Here's how the part is built. I have some questions about the finished solid (model axes, mm). A direction names the side the tool comes from. Give positions to 0.01 mm unless a question says otherwise; leave off trailing zeros. Loops run counter-clockwise (first coordinate to the right, second up) from the corner with the lowest first, then second, coordinate; pieces in that order, holes last. Notation, with made-up numbers: (50, -0.75) -> (60, -0.75) arc R14 cw to (60, 3.25) -> close; hole circle Ø4 at (66.25, 13.25). An arc over 180 degrees is marked (long way). Answer in a Markdown table with one row per item. Add a question column.
Item 1: If we section it at D-D (x = -52): Write out the boundary of the cut face in (y, z), then the cut area to 3 significant figures.
Item 2: For P1, Ø5, axis at x = -53.5, z = 2, coming from the -Y side; P2, Ø3, axis at x = -10, z = 3, coming from the +Y side; P3, Ø2.5, axis at x = -5, z = 5, coming from the +Y side, each with a flat end and sliding along its axis, tell me the tip position at first contact or that it passes through.
Item 3: If I drill on line 1 (Z direction, x = -5, y = 3.5); line 2 (Y direction, x = -12.5, z = 8.5); line 3 (Z direction, x = -47.5, y = 5.75), over which ranges is the centre line in solid material (lowest first)?
Item 4: Which directions (+Z, -Z, +X, -X, +Y, -Y) give clear straight access to the entire face, cutting with the end or side of a thin tool? Please do faces 4 (the face through (0, 3, 5)), 5 (the face through (-18, 5, 5)).
Item 5: If we section it at C-C (z = 7.75): Write out the boundary of the cut face in (x, y).
Item 6: If we section it at A-A (x = -30): Write out the boundary of the cut face in (y, z).
Item 7: We'd pull the mould along X, two halves only. Please class faces 1 (the face through (-37.95, 5.22, 4.93)), 2 (the face through (-35.7, 4.7, 0)), 3 (the face through (-63.728, 10.31, 5.601)): released by +X, released by -X, zero draft, split by the parting line, or undercut.
Item 8: If we section it at B-B (z = 4.25): Write out the boundary of the cut face in (x, y), then the cut area to 3 significant figures.
Autodesk Inventor part; units mm, degrees
ref_plane "YZ Plane" through (0, 0, 0) normal (1, 0, 0) x (0, 1, 0)
ref_plane "XZ Plane" through (0, 0, 0) normal (0, 1, 0) x (-1, 0, 0)
ref_plane "XY Plane" through (0, 0, 0) normal (0, 0, 1) x (1, 0, 0)
sketch "スケッチ1" plane through (0, 0, 0) normal (0, 0, 1) x (1, 0, 0)
  line L0 (0, 0) -> (-35, 0)
  line L1 (-35, 0) -> (-35, 5)
  line L2 (-35, 5) -> (0, 5)
  line L3 (0, 5) -> (0, 0)
  arc A0 (-42.3998, 1.1202) -> (-35, 0) centre (-35, 25) ccw
  arc A1 (-40.9198, 5.8962) -> (-35, 5) centre (-35, 25) ccw
  line L4 (-40.9198, 5.8962) -> (-42.3998, 1.1202)
  line L5 (-40.9198, 5.8962) -> (-69.5756, 14.776)
  line L6 (-69.5756, 14.776) -> (-71.0555, 10)
  line L7 (-71.0555, 10) -> (-42.3998, 1.1202)
  dimension "d3" = 5
  dimension "d4" = 5
  dimension "d6" = 20
  dimension "d7" = 35
  dimension "d8" = 10
  dimension "d23" = 30
extrude "押し出し1" add sketch "スケッチ1" along normal blind 10
sketch "スケッチ2" plane through (-42.3998, 1.1202, 0) normal (-0.295992, -0.9551904, 0) x (0.9551904, -0.295992, 0)
  line L0 (-30, 0) -> (0, 0)
  line L1 (0, 0) -> (0, 10)
  line L2 (-30, 10) -> (0, 10)
  line L3 (-30, 0) -> (-30, 10)
  circle A0 centre (-25, 5) radius 2
  circle A1 centre (-5, 5) radius 2
  point P0 (40.8315, 0)
  point P1 (0, 5)
  point P2 (-30, 5)
  dimension "d11" = 4
  dimension "d12" = 4
  dimension "d13" = 5
  dimension "d14" = 5
extrude "押し出し2" cut sketch "スケッチ2" against normal through all contours A0 | A1
sketch "スケッチ3" plane through (-35, 0, 0) normal (0, -1, 0) x (1, 0, 0)
  line L0 (0, 0) -> (35, 0)
  line L1 (35, 0) -> (35, 10)
  line L2 (0, 10) -> (35, 10)
  line L3 (0, 0) -> (0, 10)
  circle A0 centre (5, 5) radius 2
  circle A1 centre (30, 5) radius 2
  point P0 (35, 5)
  point P1 (0, 5)
  dimension "d17" = 4
  dimension "d18" = 4
  dimension "d19" = 5
  dimension "d20" = 5
extrude "押し出し3" cut sketch "スケッチ3" against normal through all contours A0 | A1
properties part number "カウンター根本1" material "アルミニウム 6061"
Recorded:
| question | item | result |
|---|---|---|
| 1 | outline | (4.1, 0) -> (9.33, 0) -> (9.33, 10) -> (4.1, 10) -> close |
| 1 | area | 52.3 mm^2 |
| 2 | P1 | stops at y = 3.79 |
| 2 | P2 | stops at y = 5 |
| 2 | P3 | passes through |
| 3 | line 1 | z = 0 to 3, 7 to 10 |
| 3 | line 2 | y = 0 to 5 |
| 3 | line 3 | z = 0 to 3.43, 6.57 to 10 |
| 4 | face 4 | +Z, -Z, +X, +Y, -Y |
| 4 | face 5 | +Z, -Z, +X, +Y |
| 5 | outline | (-71.06, 10) -> (-42.4, 1.12) arc R25 ccw to (-35, 0) -> (0, 0) -> (0, 5) -> (-35, 5) arc R20 cw to (-40.92, 5.9) -> (-69.58, 14.78) -> close |
| 6 | outline | (0, 0) -> (5, 0) -> (5, 3) -> (0, 3) -> close; (0, 7) -> (5, 7) -> (5, 10) -> (0, 10) -> close |
| 7 | face 1 | released by +X |
| 7 | face 2 | zero draft |
| 7 | face 3 | undercut |
| 8 | outline | (-71.06, 10) -> (-68.05, 9.07) -> (-66.57, 13.84) -> (-69.58, 14.78) -> close; (-64.51, 7.97) -> (-48.95, 3.15) -> (-47.47, 7.92) -> (-63.03, 12.75) -> close; (-45.4, 2.05) -> (-42.4, 1.12) arc R25 ccw to (-35, 0) -> (-31.85, 0) -> (-31.85, 5) -> (-35, 5) arc R20 cw to (-40.92, 5.9) -> (-43.92, 6.83) -> close; (-28.15, 0) -> (-6.85, 0) -> (-6.85, 5) -> (-28.15, 5) -> close; (-3.15, 0) -> (0, 0) -> (0, 5) -> (-3.15, 5) -> close |
| 8 | area | 285 mm^2 |
